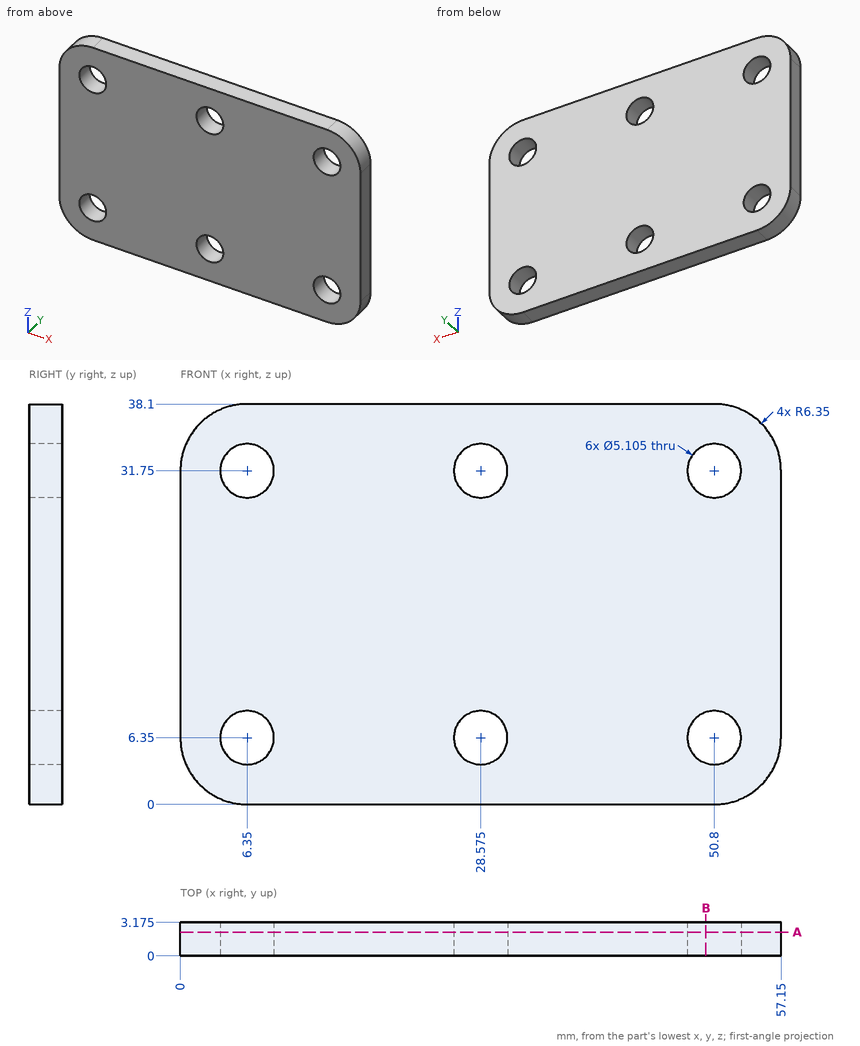
Geometry: see drawing. Coordinates: mm, zero at the bounding-box minimum. Coordinates: 2 decimals unless noted, no trailing zeros. Order: outer loops, then holes, each group sorted by start corner. A loop starts at its lowest first (then second) coordinate and runs counter-clockwise, first axis right, second up. Notation, with made-up numbers: (53.5, 13.5) - (67.5, 13.5) arc R18 cw to (67.5, 36.5) - close; hole circle Ø5 at (-34, -35). An arc over 180 degrees is marked (long way). Use one line per item in the form item = value.
1) Section A-A (y = 2.25). State how many separate pieces and enclosed holes the cut face has, then the cut area to 3 significant figures.
Solutions:
separate_pieces = 1
enclosed_holes = 6
area = 2,020 mm^2
2) Ray query, L1, parallel to X at y = 1.45, z = 31.75; L2, parallel to Z at x = 6.35, y = 1.05; L3, parallel to X at y = 1.2, z = 7. Return the intervals inside material, ascending.
Solutions:
L1 = 0 to 3.8, 8.9 to 26.02, 31.13 to 48.25, 53.35 to 57.15
L2 = 0 to 3.8, 8.9 to 29.2, 34.3 to 38.1
L3 = 0 to 3.88, 8.82 to 26.11, 31.04 to 48.33, 53.27 to 57.15
3) Section B-B (x = 50). Return loops of the section in (y, z) (1 decimal).
Solutions:
outline = (0, 0) - (3.2, 0) - (3.2, 3.9) - (0, 3.9) - close; (0, 8.8) - (3.2, 8.8) - (3.2, 29.3) - (0, 29.3) - close; (0, 34.2) - (3.2, 34.2) - (3.2, 38.1) - (0, 38.1) - close
